from build123d import *

# Parameters (mm, degrees)
F0_W     = 50
F0_H     = 25
F1_DEPTH = 25
F3_DEPTH = 25
F4_R     = 20
F5_DEPTH = 7.5
F7_DEPTH = 50.001


with BuildPart() as f1:
    # F0 (on Front) → F1 (new body, symmetric)
    with BuildSketch(Plane.XZ):
        with Locations((0, 12.5)):
            Rectangle(F0_W, F0_H)
    extrude(amount=F1_DEPTH, both=True)

    # F2 (on face) → F3 (cut)
    with BuildSketch(Plane.YZ.offset(25)):
        with BuildLine():
            Line((-2.5, 0), (2.5, 0))
            ThreePointArc((2.5, 0), (0, 2.5), (-2.5, 0))
        make_face()
    extrude(amount=-F3_DEPTH, mode=Mode.SUBTRACT)

    # F4 (on Front) → F5 (cut, symmetric)
    with BuildSketch(Plane.XZ):
        Circle(F4_R)
    extrude(amount=F5_DEPTH, both=True, mode=Mode.SUBTRACT)

    # F6 (on face) → F7 (cut, through all)
    with BuildSketch(Plane.XZ.offset(25)):
        with BuildLine():
            Line((-12, 0), (12, 0))
            ThreePointArc((12, 0), (0, 12), (-12, 0))
        make_face()
    extrude(amount=-F7_DEPTH, mode=Mode.SUBTRACT)


solid = f1.part
Verification items for the finished model (mm, model axes). A direction names the side the tool comes from. Coordinates: 2 decimals unless noted, no trailing zeros. Order: outer loops, then holes, each group sorted by start corner. A loop starts at its lowest first (then second) coordinate and runs counter-clockwise, first axis right, second up. Notation, with made-up numbers: M 73,53 L 88,53 A33 ccw 88,92 Z; hole C 83,29 d7. An arc over 180 degrees is marked long. One line per item, written item: value. Start each with the question number.
Item 1: Sectioned sample at D-D (z = 17). Enter the section's corners in (x, y).
Item 2: Scan lines: probe 1 along Y at (x, z) = (1.5, 18); probe 2 along X at (y, z) = (-4.5, 10.5); probe 3 along X at (y, z) = (21, 9.75). Record each from-to range of solid material in increasing order.
Item 3: Sectioned sample at B-B (y = 0). Enter the section's corners in (x, z).
Item 4: Sectioned sample at C-C (x = 0). Enter the section's corners in (y, z).
Item 5: Sectioned sample at A-A (z = 13.25). Enter the section's corners in (x, y).
Item 6: Gauge pin test, flat end, axial feed: pin 1 (3 mm diameter, centred on x = 9, y = 4.5, fed in from -Z). Record the tip position at first contact, or that the pin passes through.
Item 7: Mould release check, pull along X, two halves, no side actions. Record for faces 4 (the flat face through (18, 16, 0)), 5 (the flat face through (25, 0, 12)), 6 (the flat face through (-25, 0, 12)), 7 (the flat face through (-0.3, 7.5, 12.4)): released by +X, released by -X, zero draft, split by the parting line, or undercut.
Item 8: Access from +Z, -Z, +X, -X, +Y, -Y to the whole of each face (thin tool, end or side, straight path). Record for faces 1 (the flat face through (0, 0, 25)), 2 (the cylindrical face through (22.5, 0.1, 2.5)), 3 (the cylindrical face through (0, 0, 20)).
Conclusion:
1. outline: M -25,-25 L 25,-25 L 25,25 L -25,25 Z; hole M -10.54,-7.5 L 10.54,-7.5 L 10.54,7.5 L -10.54,7.5 Z
2. probe 1: y = -25 to -7.5, 7.5 to 25
2. probe 2: x = -25 to -17.02, 17.02 to 25
2. probe 3: x = -25 to -7, 7 to 25
3. outline: M -25,0 L -20,0 A20 cw 19.84,2.5 L 25,2.5 L 25,25 L -25,25 Z
4. outline: M -25,12 L -7.5,12 L -7.5,20 L 7.5,20 L 7.5,12 L 25,12 L 25,25 L -25,25 Z
5. outline: M -25,-25 L 25,-25 L 25,25 L -25,25 Z; hole M -14.98,-7.5 L 14.98,-7.5 L 14.98,7.5 L -14.98,7.5 Z
6. pin 1: stops at z = 17.02
7. face 4: zero draft
7. face 5: released by +X
7. face 6: released by -X
7. face 7: undercut
8. face 1: +Z, +X, -X, +Y, -Y
8. face 2: -Z, +X
8. face 3: -Z
